Input: part model. Units: mm. Frame: model coordinates. Face numbers are marked on the shaded views. A direction names the side the tool comes from. Coordinates: 2 decimals unless noted, no trailing zeros. Use CSV: the item, a comma, the result in double quotes.
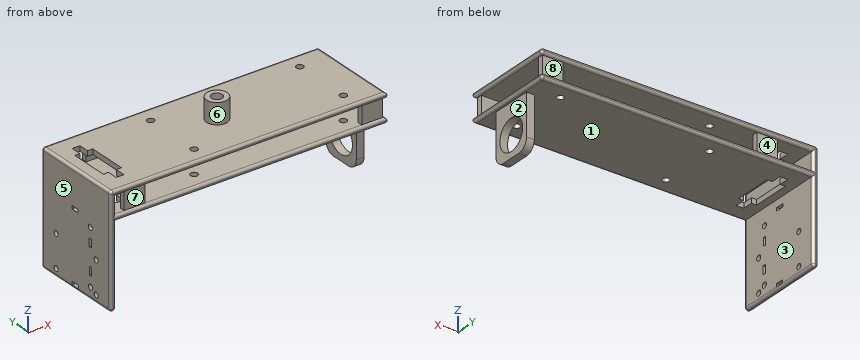
```python
from build123d import *

# Parameters (mm, degrees)
F0_W      = 105
F0_H      = 2
F1_DEPTH  = 18
F2_R      = 4
F3_DEPTH  = 8
F4_R      = 2.1
F5_DEPTH  = 3.5
F6_R      = 1.05
F7_DEPTH  = 2
F8_R      = 1.375
F9_DEPTH  = 11
F10_W     = 3
F10_H     = 4
F11_DEPTH = 11
F12_R     = 0.99999
F13_W     = 3
F13_H     = 16
F14_DEPTH = 20
F15_R     = 4
F16_R     = 6
F17_DEPTH = 3
F18_W     = 1.2
F18_H     = 3.2
F18_W_2   = 3.2
F18_H_2   = 1.2
F18_R     = 1.05
F19_DEPTH = 2
F20_W     = 8
F20_H     = 2
F21_DEPTH = 11


# Not quite as in the source:
# - a fillet or chamfer is up to 0.001 mm smaller than in the source, because OpenCascade refuses the exact size


with BuildPart() as f1:
    # F0 (on Front) → F1 (new body, symmetric)
    with BuildSketch(Plane.XZ):
        Polygon((0, -2), (0, 0), (-2, 0), (-2, -43), (0, -43), (0, -11), (0, -9), align=None)
        with Locations((52.5, -1)):
            Rectangle(F0_W, F0_H)
        with Locations((52.5, -10)):
            Rectangle(F0_W, F0_H)
    extrude(amount=F1_DEPTH, both=True)

    # F2 (on face) → F3 (join)
    with BuildSketch(Plane.XY):
        with Locations((52.5, 0)):
            Circle(F2_R)
    extrude(amount=F3_DEPTH)

    # F4 (on face) → F5 (cut)
    with BuildSketch(Plane.XY.offset(8)):
        with Locations((52.5, 0)):
            Circle(F4_R)
    extrude(amount=-F5_DEPTH, mode=Mode.SUBTRACT)

    # F6 (on face) → F7 (cut, through all)
    with BuildSketch(Plane(origin=(-2, 0, 0), x_dir=(0, -1, 0), z_dir=(-1, 0, 0))):
        with Locations((-10.5, -40)):
            Circle(F6_R)
        with Locations((10.5, -40)):
            Circle(F6_R)
        with Locations((-10.5, -27.5)):
            Circle(F6_R)
        with Locations((10.5, -27.5)):
            Circle(F6_R)
    extrude(amount=-F7_DEPTH, mode=Mode.SUBTRACT)

    # F8 (on face) → F9 (cut, through all)
    with BuildSketch(Plane.XY):
        with Locations((35.25, 11.375)):
            Circle(F8_R)
        with Locations((35.25, -11.375)):
            Circle(F8_R)
        with Locations((93, 11.375)):
            Circle(F8_R)
        with Locations((93, -11.375)):
            Circle(F8_R)
    extrude(amount=-F9_DEPTH, mode=Mode.SUBTRACT)

    # F10 (on face) → F11 (cut, through all)
    with BuildSketch(Plane.XY):
        Polygon((5, 7.5), (3, 7.5), (3, -7.5), (5, -7.5), (8, -7.5), (10, -7.5), (10, 7.5), (8, 7.5), (6.5, 7.5), align=None)
        Polygon((5, 11.5), (5, 7.5), (6.5, 7.5), (8, 7.5), (8, 11.5), align=None)
        with Locations((6.5, -9.5)):
            Rectangle(F10_W, F10_H)
    extrude(amount=-F11_DEPTH, mode=Mode.SUBTRACT)

    # F12 (radius 1 in the source; OpenCascade refuses exactly that, so slightly less here)
    f12_edges = [f1.edges().sort_by_distance(p)[0] for p in [
        (-2, 0, 0),
        (51.5, -18, 0),
        (51.5, 18, 0),
        (105, 0, 0),
        (105, 0, -2),
        (105, 0, -9),
        (105, 0, -11),
        (52.5, -18, -9),
        (52.5, -18, -11),
        (52.5, -18, -2),
        (0, -18, -27),
        (-2, -18, -21.5),
        (0, 0, -43),
        (-1, -18, -43),
        (52.5, 18, -2),
        (52.5, 18, -9),
        (52.5, 18, -11),
        (105, 18, -1),
        (105, 18, -10),
        (0, 18, -27),
        (0, 18, -5.5),
        (-2, 18, -21.5),
        (-1, 18, -43),
        (-2, 0, -43),
        (0, -18, -5.5),
    ]]
    fillet(f12_edges, radius=F12_R)

    # F13 (on face) → F14 (join)
    with BuildSketch(Plane(origin=(0, 0, -11), x_dir=(1, 0, 0), z_dir=(0, 0, -1))):
        with Locations((102, 0)):
            Rectangle(F13_W, F13_H)
    extrude(amount=F14_DEPTH)

    # F15
    f15_edges = [f1.edges().sort_by_distance(p)[0] for p in [
        (102, -8, -31),
        (102, 8, -31),
    ]]
    fillet(f15_edges, radius=F15_R)

    # F16 (on face) → F17 (cut, through all)
    with BuildSketch(Plane.YZ.offset(103.5)):
        with Locations((0, -22.608)):
            Circle(F16_R)
    extrude(amount=-F17_DEPTH, mode=Mode.SUBTRACT)

    # F18 (on face) → F19 (cut, through all)
    with BuildSketch(Plane.YZ):
        with Locations((-7.45, -22.9)):
            Rectangle(F18_W, F18_H)
        with Locations((-7.55, -32.9)):
            Rectangle(F18_W, F18_H)
        with Locations((0.45, -41.4)):
            Rectangle(F18_W_2, F18_H_2)
        with Locations((0.55, -14.4)):
            Rectangle(F18_W_2, F18_H_2)
        with Locations((-7.45, -17.3)):
            Circle(F18_R)
        with Locations((-7.55, -38.5)):
            Circle(F18_R)
    extrude(amount=-F19_DEPTH, mode=Mode.SUBTRACT)

    # F20 (on face) → F21 (join, through all)
    with BuildSketch(Plane.XY):
        with Locations((17, 16)):
            Rectangle(F20_W, F20_H)
        with Locations((100, 16)):
            Rectangle(F20_W, F20_H)
        with Locations((100, -16)):
            Rectangle(F20_W, F20_H)
        with Locations((8, -16)):
            Rectangle(F20_W, F20_H)
    extrude(amount=-F21_DEPTH)


solid = f1.part
```
(1) Ray query, probe 1 along Y at (x, z) = (93, -0.9); probe 2 along X at (y, z) = (-15.5, -6); probe 3 along Z at (x, y) = (-1.1, -10.5). Return the intervals inside material, ascending. Write a range as from..to.
Check values:
probe 1,"-17.99..-12.75, -10..10, 12.75..17.99"
probe 2,"-2..0, 4..12, 96..104"
probe 3,"-42.99..-41.05, -38.95..-28.55, -26.45..-0.01"
(2) Draft query along X for the marked faces 1, 2, 3 and 4. Return one class per face: pulls with the +X half, pulls with the -X half, needs draft (parallel to the pull), parting line crosses it, or undercut.
Check values:
face 1,"undercut"
face 2,"pulls with the +X half"
face 3,"undercut"
face 4,"needs draft"
(3) Reachability of the marked faces 5, 6, 7 and 8 from +Z, -Z, +X, -X, +Y, -Y: full face, straight path, thin tool, end or side. Return the list, or none.
Check values:
face 5,"+Z, -Z, -X, +Y, -Y"
face 6,"+Z"
face 7,"+X, -Y"
face 8,"+X, +Y"
(4) Pin query (flat end, axial travel): pin 1 Ø8 at (x, y) = (23.5, 7) entering from +Z; pin 2 Ø17 at (x, y) = (69.5, 3.5) entering from -Z; pin 3 Ø5.5 at (x, z) = (98.5, -5) entering from +Y. Return the tip coordinate at first contact, or that it passes through.
Check values:
pin 1,"z = 0"
pin 2,"z = -11"
pin 3,"y = 17"
(5) Cut plane A-A on x = 6. State how many separate pieces and enclosed holes the cut face has, and give its area (3 significant figures).
Check values:
separate pieces,"3"
enclosed holes,"0"
area,"64.3 mm^2"
